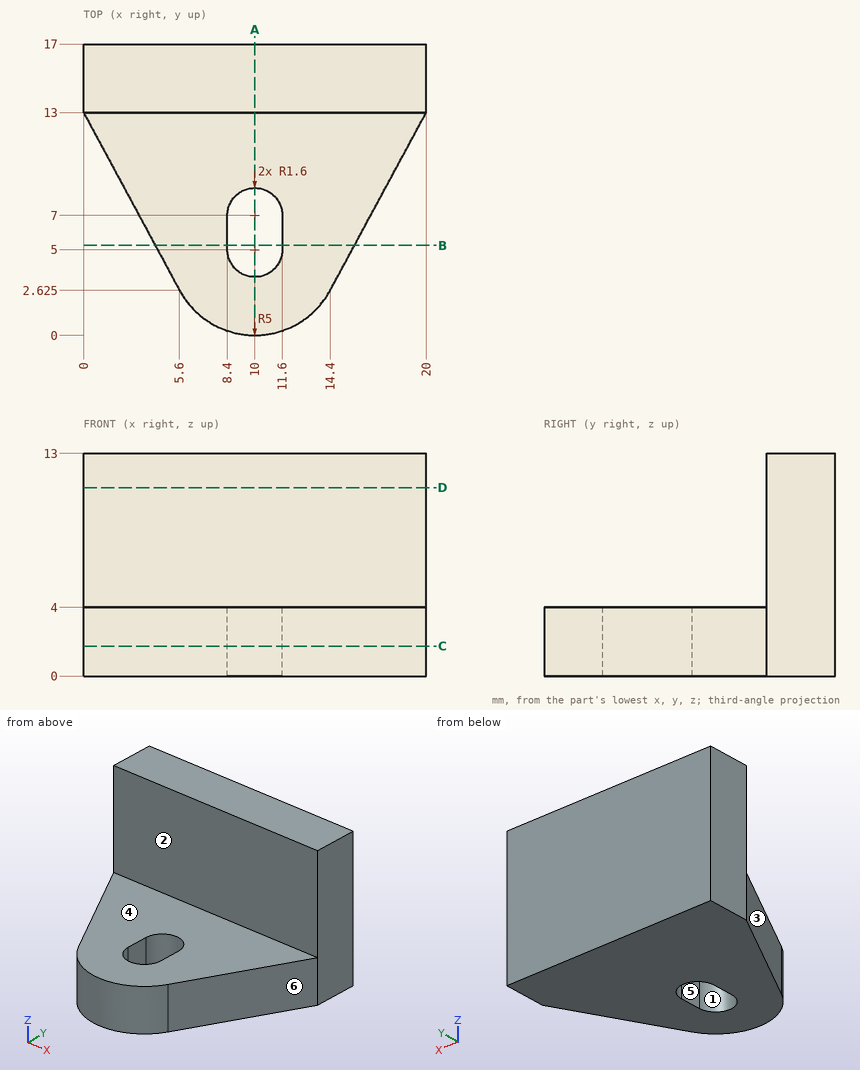
Verification items for this drawing (mm, ordinates from the low corner). A direction names the side the tool comes from. Give positions to 0.01 mm unless a question says otherwise; leave off trailing zeros. Write each loop counter-clockwise with the first axis right and the second up, starting at its lowest first coordinate (ties: lowest second). Pieces come first, ordered by that corner, then holes. Notation, with made-up numbers: M 56.5,46.25 L 108.5,46.25 A23 ccw 108.5,68.25 Z; hole C 56.5,14.5 d4. An arc over 180 degrees is marked long. Use one line per item in the form item = value.
(1) Draft check along X on the marked faces 1, 2 and 3. Enter one of: pulls with the +X half, pulls with the -X half, needs draft (parallel to the pull), parting line crosses it, or undercut.
Answer block:
face_1 = undercut
face_2 = needs draft
face_3 = pulls with the -X half
(2) Section check C-C on z = 1.75. Record the boundary of the cut face in (x, y) (3 decimals).
Answer block:
outline = M 0,13 L 5.6,2.625 A5 ccw 14.4,2.625 L 20,13 L 20,17 L 0,17 Z; hole M 8.4,5 A1.6 ccw 11.6,5 L 11.6,7 A1.6 ccw 8.4,7 Z
(3) Material ranges on line 1 along Y through (x, z) = (5.5, 5); line 2 along Z through (x, y) = (14, 9.25); line 3 along X through (y, z) = (10, 2.25), recorded low to high.
Answer block:
line_1 = 13 to 17
line_2 = 0 to 4
line_3 = 1.62 to 18.38
(4) Tool access check on the marked faces 4, 5 and 6. Record the directions out of +Z, -Z, +X, -X, +Y, -Y that give a thin tool (end or side, any length) a straight path to the whole face; none if there is none.
Answer block:
face_4 = +Z, +X, -X, -Y
face_5 = +Z, -Z
face_6 = +Z, -Z, +X, -Y
(5) Section check A-A on x = 10. Record the boundary of the cut face in (y, z).
Answer block:
outline = M 0,0 L 3.4,0 L 3.4,4 L 0,4 Z; M 8.6,0 L 17,0 L 17,13 L 13,13 L 13,4 L 8.6,4 Z
(6) Section check B-B on y = 5.25. Record the boundary of the cut face in (x, z).
Answer block:
outline = M 4.18,0 L 8.4,0 L 8.4,4 L 4.18,4 Z; M 11.6,0 L 15.82,0 L 15.82,4 L 11.6,4 Z
(7) Depth check by flat-ended pin: P1, Ø6, axis at y = 7, z = 4, coming from the -X side; P2, Ø0.6, axis at y = 6, z = 2.5, coming from the +X side; P3, Ø3, axis at x = 15.5, z = 10, coming from the -Y side; P4, Ø5, axis at y = 2.5, z = 7.5, coming from the -X side. Enter the tip coordinate at first touch or a pass-through.
Answer block:
P1 = 1.62
P2 = 16.38
P3 = 13
P4 = through
(8) Section check D-D on z = 11. Record the boundary of the cut face in (x, y), plus the area to 3 significant figures.
Answer block:
outline = M 0,13 L 20,13 L 20,17 L 0,17 Z
area = 80.0 mm2
